Design review of the part shown in the three views and the two pictorial views. Dimensions are in mm from the part's minimum x, y and z. Round coordinates to 2 decimals unless told otherwise and drop trailing zeros. Order: outer loops, then holes, each group sorted by start corner. A loop starts at its lowest first (then second) coordinate and runs counter-clockwise, first axis right, second up. Notation, with made-up numbers: (-1, 63.5) - (26, 63.5) arc R30 cw to (26, 97.5) - close; hole circle Ø2 at (-8, 72.25). An arc over 180 degrees is marked (long way). One line per question, with ' | ' between items. Start each with the question number.
Item 1: Insertion check: pin 1 Ø8 at (x, z) = (306, 16.5) entering from -Y; pin 2 Ø4 at (y, z) = (137, 17.5) entering from -X; pin 3 Ø6 at (y, z) = (451.5, 9.5) entering from -X. Each pin has a flat end and moves straight along its axis. Give the tip position at first contact, or say it passes through.
Item 2: Add section C-C on y = 521. State the section outline as (x, z) points, and give its area (3 significant figures).
Item 3: For L1, parallel to X at y = 141, z = 22; L2, parallel to Y at x = 257.5, z = 17.25; L3, parallel to Y at x = 231.5, z = 14, list the stretches that pass through material, from the lowest coordinate up. Write a range as [from, to].
Item 4: Add section A-A on z = 18.75. State the section outline as (x, y) points (1 decimal).
Item 5: Add section B-B on x = 261. State the section outline as (y, z) points, and give its area (3 significant figures).
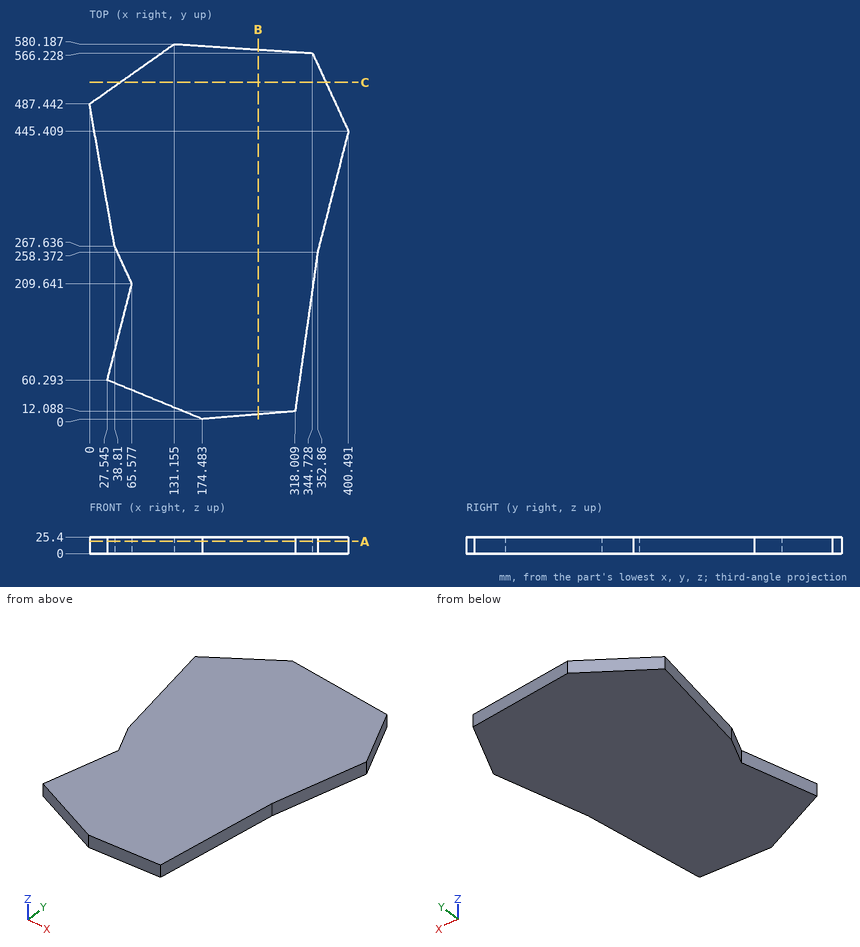
Determined:
1) pin 1: y = 10.74 | pin 2: x = 46.57 | pin 3: x = 5.82
2) outline: (47.46, 0) - (365.6, 0) - (365.6, 25.4) - (47.46, 25.4) - close | area: 8,080 mm2
3) L1: [48.1, 336.25] | L2: [6.99, 571.93] | L3: [4.8, 573.63]
4) outline: (0, 487.4) - (38.8, 267.6) - (65.6, 209.6) - (27.5, 60.3) - (174.5, 0) - (318, 12.1) - (352.9, 258.4) - (400.5, 445.4) - (344.7, 566.2) - (131.2, 580.2) - close
5) outline: (7.29, 0) - (571.7, 0) - (571.7, 25.4) - (7.29, 25.4) - close | area: 14,300 mm2
